from build123d import *

# Parameters (mm, degrees)
F0_R     = 14.224
F1_DEPTH = 31.75
F2_R     = 9.652
F3_DEPTH = 19.05
F5_D     = 3.7973
F7_DEPTH = 31.75
F8_R     = 3.2512
F9_DEPTH = 25.401


with BuildPart() as f1:
    # F0 (on Top) → F1 (new body)
    with BuildSketch(Plane.XY):
        Circle(F0_R)
    extrude(amount=F1_DEPTH)

    # F2 (on face) → F3 (cut)
    with BuildSketch(Plane(origin=(0, 0, 0), x_dir=(1, 0, 0), z_dir=(0, 0, -1))):
        Circle(F2_R)
    extrude(amount=-F3_DEPTH, mode=Mode.SUBTRACT)

    # F5 (through all)
    with Locations(Plane.XY.offset(31.75)):
        with Locations((0, 0)):
            Hole(F5_D / 2)

    # F6 (on face) → F7 (cut, through all)
    with BuildSketch(Plane.XY.offset(31.75)):
        with BuildLine():
            Line((-12.7, -6.4056362682), (-12.7, 6.4056362682))
            ThreePointArc((-12.7, 6.4056362682), (-14.224, 0), (-12.7, -6.4056362682))
        make_face()
        with BuildLine():
            ThreePointArc((12.7, -6.4056362682), (14.224, 0), (12.7, 6.4056362682))
            Line((12.7, 6.4056362682), (12.7, -6.4056362682))
        make_face()
    extrude(amount=-F7_DEPTH, mode=Mode.SUBTRACT)

    # F8 (on face) → F9 (cut, through all)
    with BuildSketch(Plane.YZ.offset(12.7)):
        with Locations((0, 22.86)):
            Circle(F8_R)
    extrude(amount=-F9_DEPTH, mode=Mode.SUBTRACT)


solid = f1.part
Here's how the part is built. I have some questions about the finished solid (model axes, mm). A direction names the side the tool comes from. Coordinates: 2 decimals unless noted, no trailing zeros. Order: outer loops, then holes, each group sorted by start corner. A loop starts at its lowest first (then second) coordinate and runs counter-clockwise, first axis right, second up. Notation, with made-up numbers: M 84.25,9 L 110.25,9 A23 cw 110.25,43 Z; hole C 23,6 d2. An arc over 180 degrees is marked long. Answer as CSV lines item,"result".
Item 1: Imagine slicing it at A-A on y = 0. Write out the boundary of the cut face in (x, z).
Results found:
outline,"M -12.7,0 L -9.65,0 L -9.65,19.05 L -1.9,19.05 L -1.9,19.61 L -12.7,19.61 Z; M -12.7,26.11 L -1.9,26.11 L -1.9,31.75 L -12.7,31.75 Z; M 1.9,19.05 L 9.65,19.05 L 9.65,0 L 12.7,0 L 12.7,19.61 L 1.9,19.61 Z; M 1.9,26.11 L 12.7,26.11 L 12.7,31.75 L 1.9,31.75 Z"
Item 2: We'd pull the mould along Y, two halves only. Please class faces 1 (the face through (0.22, 14.222, 15.653)), 2 (the face through (12.7, 0, 16)), 3 (the face through (-2.3, -0.1, 19.05)): +Y half, -Y half, draft (parallel to the pull), parting line (faces both ways), or undercut.
Results found:
face 1,"+Y half"
face 2,"draft"
face 3,"undercut"
Item 3: Imagine slicing it at C-C on x = 0. Write out the boundary of the cut face in (y, z), plus the area to 3 significant figures.
Results found:
outline,"M -14.22,0 L -9.65,0 L -9.65,19.05 L -1.9,19.05 L -1.9,20.22 A3.25 cw -1.9,25.5 L -1.9,31.75 L -14.22,31.75 Z; M 1.9,19.05 L 9.65,19.05 L 9.65,0 L 14.22,0 L 14.22,31.75 L 1.9,31.75 L 1.9,25.5 A3.25 cw 1.9,20.22 Z"
area,"477 mm2"
Item 4: Imagine slicing it at D-D on z = 30. Write out the boundary of the cut face in (x, y), plus the area to 3 significant figures.
Results found:
outline,"M -12.7,-6.41 A14.22 ccw 12.7,-6.41 L 12.7,6.41 A14.22 ccw -12.7,6.41 Z; hole C 0,0 d3.8"
area,"598 mm2"
Item 5: Imagine slicing it at B-B on z = 22.86. Write out the boundary of the cut face in (x, y).
Results found:
outline,"M -12.7,-6.41 A14.22 ccw 12.7,-6.41 L 12.7,-3.25 L -12.7,-3.25 Z; M -12.7,3.25 L 12.7,3.25 L 12.7,6.41 A14.22 ccw -12.7,6.41 Z"
Item 6: On a 3-axis mill with a long thin cutter (end or side, diameter ignored), from which of +Z, -Z, +X, -X, +Y, -Y can I reach the whole of each face in a straight line? I mean faces 4 (the face through (-7.66, 5.87, 9.39)), 5 (the face through (0, 10, 0)). Say none if no direction works.
Results found:
face 4,"-Z"
face 5,"-Z, +X, -X, +Y, -Y"
Item 7: For pin 1 (12 mm diameter, centred on x = -7, z = 16.5, fed in from +Y); pin 2 (5 mm diameter, centred on x = 0, y = 0, fed in from -Z); pin 3 (10 mm diameter, centred on x = -1.5, y = 0.5, fed in from +Z); pin 4 (1 mm diameter, centred on x = -5, z = 6.5, fed in from -Y), each with a flat end and sliding along its axis, tell me the tip position at first contact or that it passes through.
Results found:
pin 1,"y = 14.19"
pin 2,"z = 19.05"
pin 3,"z = 31.75"
pin 4,"y = -13.49"
Item 8: If I drill on line 1 (Z direction, x = -2.75, y = 0); line 2 (Y direction, x = -8.25, z = 5); line 3 (Y direction, x = 7.5, z = 4.5), over which ranges is the centre line in solid material (lowest first)?
Results found:
line 1,"19.05 to 19.61, 26.11 to 31.75"
line 2,"-11.59 to -5.01, 5.01 to 11.59"
line 3,"-12.09 to -6.08, 6.08 to 12.09"
